from build123d import *

# Parameters (mm, degrees)
F0_W     = 63.5
F0_H     = 76.2
F1_DEPTH = 12.7
F2_W     = 12.7
F2_H     = 76.2
F3_DEPTH = 50.8
F4_W     = 5.442066
F4_H     = 25.4
F4_H_2   = 12.7
F5_DEPTH = 12.7
F6_W     = 25.4
F6_H     = 25.4
F7_DEPTH = 12.7


with BuildPart() as f1:
    # F0 (on Front) → F1 (new body)
    with BuildSketch(Plane.XZ):
        with Locations((-0.396088, 4.24908)):
            Rectangle(F0_W, F0_H)
    extrude(amount=F1_DEPTH)

    # F2 (on face) → F3 (join)
    with BuildSketch(Plane.XZ.offset(12.7)):
        with Locations((-25.796088, 4.24908)):
            Rectangle(F2_W, F2_H)
    extrude(amount=F3_DEPTH)

    # F4 (on face) → F5 (cut)
    with BuildSketch(Plane.YZ.offset(-19.446088)):
        Polygon((-38.1, 16.94908), (-63.5, 16.94908), (-63.5, 4.24908), (-58.057934, 4.24908), (-38.1, 4.24908), align=None)
        with Locations((-60.778967, -8.45092)):
            Rectangle(F4_W, F4_H)
        with Locations((-60.778967, -27.50092)):
            Rectangle(F4_W, F4_H_2)
    extrude(amount=-F5_DEPTH, mode=Mode.SUBTRACT)

    # F6 (on face) → F7 (cut)
    with BuildSketch(Plane.YZ.offset(-19.446088)):
        with Locations((-45.357934, -21.15092)):
            Rectangle(F6_W, F6_H)
    extrude(amount=-F7_DEPTH, mode=Mode.SUBTRACT)


solid = f1.part
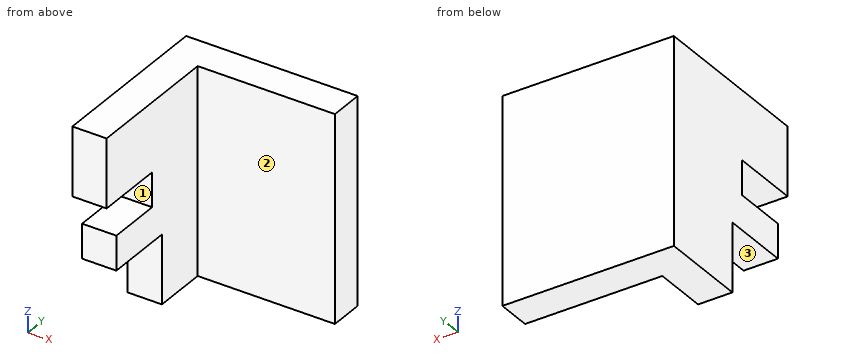
Model file for the job. Use its own axes, mm. Face numbers are marked on the shaded views. A direction names the side the tool comes from. Coordinates: 2 decimals unless noted, no trailing zeros. Write each loop counter-clockwise with the first axis right and the second up, starting at its lowest first coordinate (ties: lowest second). Pieces come first, ordered by that corner, then holes. Notation, with made-up numbers: (-38, -17.75) - (6, -17.75) arc R26 cw to (6, 10.25) - close; hole circle Ø10 at (28, 37.5). An arc over 180 degrees is marked (long way). Write each question's results on one line, items separated by ' | '. Start each with the question number.
1) Cut at D-D (y = -26.5). Write the cut outline in (x, z).
2) 3-axis set-ups, long thin cutter, end or side, ignore diameter. For the marked faces 1, 2 and 3: which of +Z, -Z, +X, -X, +Y, -Y reach the whole face in a straight line?
3) Cut at C-C (z = 14.5). Write the cut outline in (x, y).
4) Flat gauge pins, fed straight in: P1, Ø4, axis at y = -20.5, z = 24, coming from the +X side; P2, Ø6.5, axis at x = -26.5, y = -51, coming from the -Z side; P3, Ø6.5, axis at x = -24, z = 8, coming from the -Y side. Where does each tip first touch, or does it go through?
5) Cut at B-B (x = -27). Write the cut outline in (y, z), then the cut area to 3 significant figures.
6) Probe line 1 along X through (y, z) = (-13, 21.5); line 2 along Y through (x, z) = (8, -12.5); line 3 along Y through (x, z) = (-20.5, -8). List the from-to ranges inside material, lowest first. Write a range as from..to.
7) Cut at A-A (y = -52.5). Write the cut outline in (x, z), then the cut area to 3 significant figures.
Returned:
1) outline: (-32.15, -33.85) - (-19.45, -33.85) - (-19.45, 42.35) - (-32.15, 42.35) - close
2) face 1: +X, -X, -Y | face 2: +Z, -Z, +X, -Y | face 3: -Z, +X, -X, -Y
3) outline: (-32.15, -38.1) - (-19.45, -38.1) - (-19.45, -12.7) - (31.35, -12.7) - (31.35, 0) - (-32.15, 0) - close
4) P1: x = -19.45 | P2: z = -8.45 | P3: y = -38.1
5) outline: (-63.5, 16.95) - (-38.1, 16.95) - (-38.1, 4.25) - (-58.06, 4.25) - (-58.06, -8.45) - (-32.66, -8.45) - (-32.66, -33.85) - (0, -33.85) - (0, 42.35) - (-63.5, 42.35) - close | area: 3,660 mm^2
6) line 1: -32.15..-19.45 | line 2: -12.7..0 | line 3: -58.06..0
7) outline: (-32.15, -8.45) - (-19.45, -8.45) - (-19.45, 4.25) - (-32.15, 4.25) - close; (-32.15, 16.95) - (-19.45, 16.95) - (-19.45, 42.35) - (-32.15, 42.35) - close | area: 484 mm^2
